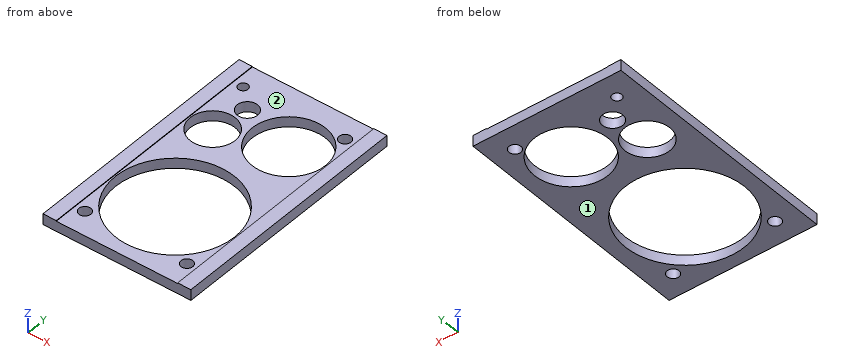
from build123d import *

# Parameters (mm, degrees)
SKETCH1_W           = 145
SKETCH1_H           = 238
SKETCH1_R           = 5.8
SKETCH1_R_2         = 22
SKETCH1_R_3         = 36
SKETCH1_R_4         = 58.25
SKETCH1_R_5         = 10
SKETCH1_R_6         = 4.75
BOSS_EXTRUDE1_DEPTH = 10
SKETCH2_W           = 13
SKETCH2_H           = 238
BOSS_EXTRUDE2_DEPTH = 0.6


with BuildPart() as part:
    # Sketch1 → Boss-Extrude1 (new body)
    with BuildSketch(Plane.XY):
        Rectangle(SKETCH1_W, SKETCH1_H)
        with Locations((50, 96)):
            Circle(SKETCH1_R, mode=Mode.SUBTRACT)
        with Locations((50, -96)):
            Circle(SKETCH1_R, mode=Mode.SUBTRACT)
        with Locations((-50, -96)):
            Circle(SKETCH1_R, mode=Mode.SUBTRACT)
        with Locations((-36.25, 42)):
            Circle(SKETCH1_R_2, mode=Mode.SUBTRACT)
        with Locations((22.25, 62)):
            Circle(SKETCH1_R_3, mode=Mode.SUBTRACT)
        with Locations((0, -48.5)):
            Circle(SKETCH1_R_4, mode=Mode.SUBTRACT)
        with Locations((-30, 76.5)):
            Circle(SKETCH1_R_5, mode=Mode.SUBTRACT)
        with Locations((-50, 96)):
            Circle(SKETCH1_R_6, mode=Mode.SUBTRACT)
    extrude(amount=BOSS_EXTRUDE1_DEPTH)

    # Sketch2 → Boss-Extrude2 (add)
    with BuildSketch(Plane.XY.offset(10)):
        with Locations((-66, 0)):
            Rectangle(SKETCH2_W, SKETCH2_H)
        with Locations((66, 0)):
            Rectangle(SKETCH2_W, SKETCH2_H)
    extrude(amount=BOSS_EXTRUDE2_DEPTH)


solid = part.part
Read the model definition and answer for the solid it produces. Units are mm, in the model's axes. Face numbers are marked on the shaded views. Give positions to 0.01 mm unless a question says otherwise; leave off trailing zeros. Write each loop counter-clockwise with the first axis right and the second up, starting at its lowest first coordinate (ties: lowest second). Pieces come first, ordered by that corner, then holes. Notation, with made-up numbers: M 36.5,55.5 L 46.5,55.5 A32 ccw 46.5,86.5 Z; hole C 3,-39 d9. An arc over 180 degrees is marked long. One line per item, written item: value. Start each with the question number.
(1) Find section D-D (y = -48.5). Determine the outline of the cut face in (x, z), plus the area to 3 significant figures.
(2) Determine the mould class of the marked faces 1 and 2 for opening direction X: pulls with the +X half, pulls with the -X half, needs draft (parallel to the pull), parting line crosses it, or undercut.
(3) Find the intervals of material crossed by line 1 (Y direction, x = 0, z = 5.5); line 2 (X direction, y = 29, z = 9.5); line 3 (Y direction, x = -36.25, z = 7.25), in increasing order.
(4) Find section A-A (y = 76.5). Determine the outline of the cut face in (x, z).
(5) Find section C-C (y = -96). Determine the outline of the cut face in (x, z), plus the area to 3 significant figures.
(6) Find section B-B (x = 50). Determine the outline of the cut face in (y, z).
(7) A flat-ended cylindrical pin translates along its axis: pin 1 Ø13.5 at (x, y) = (-50, -96) entering from +Z. Find the tip coordinate at first contact, or state that the pin passes through.
Results below:
1. outline: M -72.5,0 L -58.25,0 L -58.25,10 L -59.5,10 L -59.5,10.6 L -72.5,10.6 Z; M 58.25,0 L 72.5,0 L 72.5,10.6 L 59.5,10.6 L 59.5,10 L 58.25,10 Z
1. area: 301 mm^2
2. face 1: needs draft
2. face 2: undercut
3. line 1: y = -119 to -106.75, 9.75 to 33.7, 90.3 to 119
3. line 2: x = -72.5 to -54, -18.5 to 7.86, 36.64 to 72.5
3. line 3: y = -119 to -94.1, -2.9 to 20, 64 to 68.69, 84.31 to 119
4. outline: M -72.5,0 L -40,0 L -40,10 L -59.5,10 L -59.5,10.6 L -72.5,10.6 Z; M -20,0 L -10.7,0 L -10.7,10 L -20,10 Z; M 55.2,0 L 72.5,0 L 72.5,10.6 L 59.5,10.6 L 59.5,10 L 55.2,10 Z
5. outline: M -72.5,0 L -55.8,0 L -55.8,10 L -59.5,10 L -59.5,10.6 L -72.5,10.6 Z; M -44.2,0 L -33.72,0 L -33.72,10 L -44.2,10 Z; M 33.72,0 L 44.2,0 L 44.2,10 L 33.72,10 Z; M 55.8,0 L 72.5,0 L 72.5,10.6 L 59.5,10.6 L 59.5,10 L 55.8,10 Z
5. area: 559 mm^2
6. outline: M -119,0 L -101.8,0 L -101.8,10 L -119,10 Z; M -90.2,0 L -78.38,0 L -78.38,10 L -90.2,10 Z; M -18.62,0 L 39.07,0 L 39.07,10 L -18.62,10 Z; M 84.93,0 L 90.2,0 L 90.2,10 L 84.93,10 Z; M 101.8,0 L 119,0 L 119,10 L 101.8,10 Z
7. pin 1: stops at z = 10
